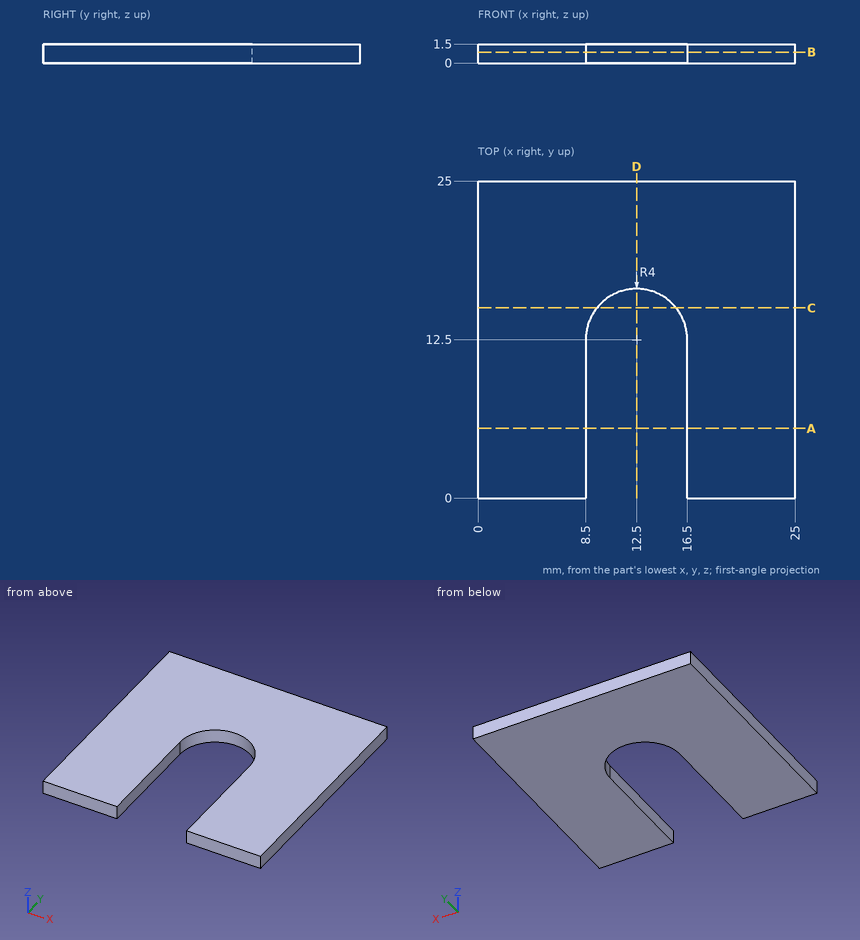
Source: three-view drawing plus pictorial views. Frame: mm from the lowest corner of the part. Coordinates: 2 decimals unless noted, no trailing zeros. Write each loop counter-clockwise with the first axis right and the second up, starting at its lowest first coordinate (ties: lowest second). Pieces come first, ordered by that corner, then holes. Notation, with made-up numbers: (48.25, 75) - (92.25, 75) arc R19 ccw to (92.25, 96) - close; hole circle Ø11 at (-38.5, -16.5). An arc over 180 degrees is marked (long way). Answer as a JSON object with one key per item and string values.
Q1. Section query C-C, the plane y = 15. Output: boundary loops of the cut face in (x, z).
Ans:
{"outline": "(0, 0) - (9.38, 0) - (9.38, 1.5) - (0, 1.5) - close; (15.62, 0) - (25, 0) - (25, 1.5) - (15.62, 1.5) - close"}
Q2. Material intervals for line 1 (X direction, y = 9, z = 0.1); line 2 (X direction, y = 14.75, z = 0.1); line 3 (Y direction, x = 10.75, z = 1.15), sorted ascending. Write a range as [from, to].
Ans:
{"line 1": "x = [0, 8.5], [16.5, 25]", "line 2": "x = [0, 9.19], [15.81, 25]", "line 3": "y = [16.1, 25]"}
Q3. Section query D-D, the plane x = 12.5. Output: boundary loops of the cut face in (y, z), plus the area to 4 significant figures.
Ans:
{"outline": "(16.5, 0) - (25, 0) - (25, 1.5) - (16.5, 1.5) - close", "area": "12.75 mm2"}
Q4. Section query A-A, the plane y = 5.5. Output: boundary loops of the cut face in (x, z), plus the area to 3 significant figures.
Ans:
{"outline": "(0, 0) - (8.5, 0) - (8.5, 1.5) - (0, 1.5) - close; (16.5, 0) - (25, 0) - (25, 1.5) - (16.5, 1.5) - close", "area": "25.5 mm2"}
Q5. Section query B-B, the plane z = 0.85. Output: boundary loops of the cut face in (x, y).
Ans:
{"outline": "(0, 0) - (8.5, 0) - (8.5, 12.5) arc R4 cw to (16.5, 12.5) - (16.5, 0) - (25, 0) - (25, 25) - (0, 25) - close"}
